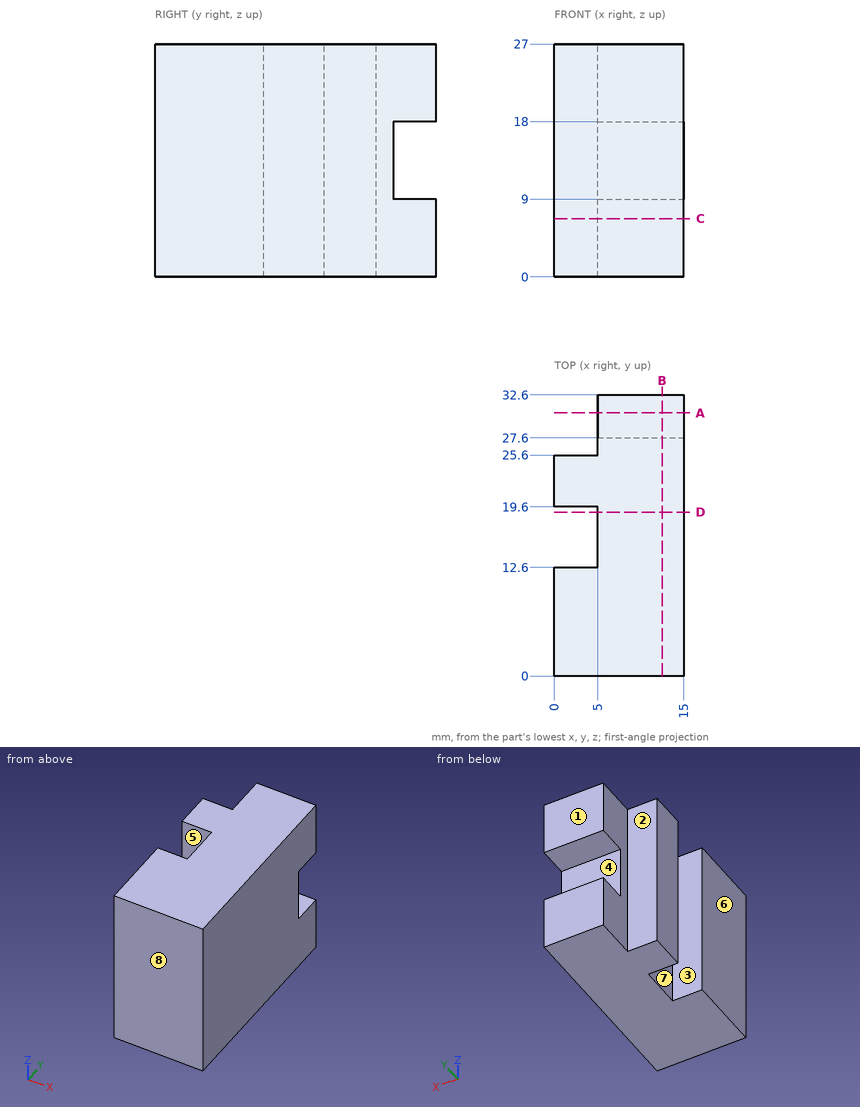
Geometry: see drawing. Coordinates: mm, zero at the bounding-box minimum. A direction names the side the tool comes from. Give positions to 0.01 mm unless a question says otherwise; leave off trailing zeros. Loops run counter-clockwise (first coordinate to the right, second up) from the corner with the lowest first, then second, coordinate; pieces in that order, holes last. Notation, with made-up numbers: (-5.75, 79) - (52.25, 79) arc R10 ccw to (52.25, 93) - close; hole circle Ø6 at (36.5, 76). An arc over 180 degrees is marked (long way). Use CSV: the item, a comma, the result in double quotes. Start each with the question number.
1. Section B-B (x = 12.5). Output: boundary loops of the cut face in (y, z).
2. Reachability of the marked faces 1, 2, 3 and 4 from +Z, -Z, +X, -X, +Y, -Y: full face, straight path, thin tool, end or side. Return the list, or none.
3. Section D-D (y = 19). Output: boundary loops of the cut face in (x, z).
4. Pin query (flat end, axial travel): pin 1 (5.5 mm diameter, centred on x = 2, z = 11, fed in from +Y); pin 2 (2.5 mm diameter, centred on x = 9, z = 14, fed in from +Y); pin 3 (7.5 mm diameter, centred on y = 30, z = 11.5, fed in from -X). Return the tip coordinate at first contact, or that it passes through.
5. Ray query, L1, parallel to Z at x = 10, y = 28; L2, parallel to Y at x = 2, z = 7.5; L3, parallel to Y at x = 12.75, z = 13. Return the intervals inside material, ascending.
6. Draft query along Y for the marked faces 5, 6, 7 and 8. Return one class per face: +Y half, -Y half, draft (parallel to the pull), parting line (faces both ways), or undercut.
7. Section A-A (y = 30.5). Output: boundary loops of the cut face in (x, z).
8. Section C-C (z = 6.75). Output: boundary loops of the cut face in (x, y), then the cut area to 3 significant figures.
Response:
1,outline,"(0, 0) - (32.6, 0) - (32.6, 9) - (27.6, 9) - (27.6, 18) - (32.6, 18) - (32.6, 27) - (0, 27) - close"
2,face 1,"+Z, -Z, +X, -X, +Y"
2,face 2,"+Z, -Z, -X, +Y"
2,face 3,"+Z, -Z, -X"
2,face 4,"+X, -X, +Y"
3,outline,"(5, 0) - (15, 0) - (15, 27) - (5, 27) - close"
4,pin 1,"y = 25.6"
4,pin 2,"y = 27.6"
4,pin 3,"x = 5"
5,L1,"0 to 9, 18 to 27"
5,L2,"0 to 12.6, 19.6 to 25.6"
5,L3,"0 to 27.6"
6,face 5,"undercut"
6,face 6,"draft"
6,face 7,"undercut"
6,face 8,"-Y half"
7,outline,"(5, 0) - (15, 0) - (15, 9) - (5, 9) - close; (5, 18) - (15, 18) - (15, 27) - (5, 27) - close"
8,outline,"(0, 0) - (15, 0) - (15, 32.6) - (5, 32.6) - (5, 25.6) - (0, 25.6) - (0, 19.6) - (5, 19.6) - (5, 12.6) - (0, 12.6) - close"
8,area,"419 mm²"
